from build123d import *

# Parameters (mm, degrees)
BOSS_EXTRU_1_DEPTH                  = 60
CHANFREIN2_SIZE                     = 10
CHANFREIN2_SIZE2                    = 20
CHANFREIN3_SIZE                     = 20
CHANFREIN3_SIZE2                    = 10
CONG_3_R                            = 2
ENL_V_MAT_EXTRU_4_DEPTH             = 2
ENL_V_MAT_EXTRU_4_DEPTH_BACK        = 66.720872054
ENL_V_MAT_EXTRU_4_START             = -4
ESQUISSE5_R                         = 16.05
ESQUISSE2_R                         = 1.7
ESQUISSE2_R_2                       = 10.1
ENL_V_MAT_EXTRU_1_DEPTH             = 70.720872183
ESQUISSE3_R                         = 1.6
ENL_V_MAT_EXTRU_2_DEPTH             = 78.097341186
ENL_V_MAT_EXTRU_5_REACH             = 71.721
ESQUISSE6_R                         = 3.25
ENL_V_MAT_EXTRU_5_DIRECTION_2_REACH = 71.721
CHANFREIN1_SIZE                     = 10
BOSS_EXTRU_3_REACH                  = 79.097
ESQUISSE8_W                         = 1.2
ESQUISSE8_H                         = 30
CONG_2_R                            = 2


with BuildPart() as part:
    # Esquisse1 → Boss.-Extru.1 (new body)
    with BuildSketch(Plane(origin=(0, 0, 0), x_dir=(0, 0, -1), z_dir=(1, 0, 0))):
        Polygon((0, -19), (0, 19), (30, 19), (30, 15), (4, 15), (4, -15), (30, -15), (30, -19), align=None)
    extrude(amount=BOSS_EXTRU_1_DEPTH)

    # Chanfrein2
    chanfrein2_edges = [part.edges().sort_by_distance(p)[0] for p in [
        (30, 15, -4),
    ]]
    chanfrein2_side = [part.faces().sort_by_distance(p)[0] for p in [
        (30, 0, -4),
    ]]
    chamfer(chanfrein2_edges, length=CHANFREIN2_SIZE, length2=CHANFREIN2_SIZE2, reference=chanfrein2_side[0])

    # Chanfrein3
    chanfrein3_edges = [part.edges().sort_by_distance(p)[0] for p in [
        (30, -15, -4),
    ]]
    chanfrein3_side = [part.faces().sort_by_distance(p)[0] for p in [
        (30, -15, -17),
    ]]
    chamfer(chanfrein3_edges, length=CHANFREIN3_SIZE, length2=CHANFREIN3_SIZE2, reference=chanfrein3_side[0])

    # Congé3
    cong_3_edges = [part.edges().sort_by_distance(p)[0] for p in [
        (30, 5, -4),
        (30, -5, -4),
    ]]
    fillet(cong_3_edges, radius=CONG_3_R)

    # Esquisse5 → Enlèv. mat.-Extru.4 (cut, two sides: drawn at the far end of the back side and taken through both)
    with BuildSketch(Plane.XY.offset(ENL_V_MAT_EXTRU_4_START - ENL_V_MAT_EXTRU_4_DEPTH_BACK)):
        with Locations(Location((30, 0, 0), (0, 0, 193.562911562))):
            Circle(ESQUISSE5_R)
    extrude(amount=ENL_V_MAT_EXTRU_4_DEPTH + ENL_V_MAT_EXTRU_4_DEPTH_BACK, mode=Mode.SUBTRACT)

    # Esquisse2 → Enlèv. mat.-Extru.1 (cut, through all)
    with BuildSketch(Plane.XY):
        with Locations((30, 13)):
            Circle(ESQUISSE2_R)
        with Locations((43, 0)):
            Circle(ESQUISSE2_R)
        with Locations((30, -13)):
            Circle(ESQUISSE2_R)
        with Locations((17, 0)):
            Circle(ESQUISSE2_R)
        with Locations((30, 0)):
            Circle(ESQUISSE2_R_2)
    extrude(amount=-ENL_V_MAT_EXTRU_1_DEPTH, mode=Mode.SUBTRACT)

    # Esquisse3 → Enlèv. mat.-Extru.2 (cut, through all)
    with BuildSketch(Plane.XZ.offset(19)):
        with Locations(Location((10, -15, 0), (0, 0, 270))):
            Circle(ESQUISSE3_R)
        with Locations(Location((50, -15, 0), (0, 0, 270))):
            Circle(ESQUISSE3_R)
    extrude(amount=-ENL_V_MAT_EXTRU_2_DEPTH, mode=Mode.SUBTRACT)

    # Enlèv. mat.-Extru.5: up to this face of the body (flat: up to its plane)
    enl_v_mat_extru_5_end = Plane(part.part.faces().sort_by_distance((30, -19, -15))[0])
    # Esquisse6 → Enlèv. mat.-Extru.5 (cut, up to the picked face)
    with BuildSketch(Plane(origin=(0, 0, 0), x_dir=(1, 0, 0), z_dir=(0, 1, 0)), mode=Mode.PRIVATE) as enl_v_mat_extru_5_sk1:
        with Locations(Location((10, 15, 0), (0, 0, 90))):
            Circle(ESQUISSE6_R)
    enl_v_mat_extru_5_tool1 = split(extrude(enl_v_mat_extru_5_sk1.sketch, amount=-ENL_V_MAT_EXTRU_5_REACH, mode=Mode.PRIVATE), bisect_by=enl_v_mat_extru_5_end, keep=Keep.BOTH, mode=Mode.PRIVATE)
    # Esquisse6 → Enlèv. mat.-Extru.5 (cut, up to the picked face)
    with BuildSketch(Plane(origin=(0, 0, 0), x_dir=(1, 0, 0), z_dir=(0, 1, 0)), mode=Mode.PRIVATE) as enl_v_mat_extru_5_sk2:
        with Locations(Location((50, 15, 0), (0, 0, 270))):
            Circle(ESQUISSE6_R)
    enl_v_mat_extru_5_tool2 = split(extrude(enl_v_mat_extru_5_sk2.sketch, amount=-ENL_V_MAT_EXTRU_5_REACH, mode=Mode.PRIVATE), bisect_by=enl_v_mat_extru_5_end, keep=Keep.BOTH, mode=Mode.PRIVATE)
    add(enl_v_mat_extru_5_tool1.solids().sort_by(Axis((10, 0, -15), (0, -1, 0)))[0], mode=Mode.SUBTRACT)
    add(enl_v_mat_extru_5_tool2.solids().sort_by(Axis((50, 0, -15), (0, -1, 0)))[0], mode=Mode.SUBTRACT)

    # Enlèv. mat.-Extru.5 direction 2: up to this face of the body (flat: up to its plane)
    enl_v_mat_extru_5_direction_2_end = Plane(part.part.faces().sort_by_distance((30, 19, -15))[0])
    # Esquisse6 → Enlèv. mat.-Extru.5 direction 2 (cut, up to the picked face)
    with BuildSketch(Plane(origin=(0, 0, 0), x_dir=(1, 0, 0), z_dir=(0, 1, 0)), mode=Mode.PRIVATE) as enl_v_mat_extru_5_direction_2_sk1:
        with Locations(Location((10, 15, 0), (0, 0, 90))):
            Circle(ESQUISSE6_R)
    enl_v_mat_extru_5_direction_2_tool1 = split(extrude(enl_v_mat_extru_5_direction_2_sk1.sketch, amount=ENL_V_MAT_EXTRU_5_DIRECTION_2_REACH, mode=Mode.PRIVATE), bisect_by=enl_v_mat_extru_5_direction_2_end, keep=Keep.BOTH, mode=Mode.PRIVATE)
    # Esquisse6 → Enlèv. mat.-Extru.5 direction 2 (cut, up to the picked face)
    with BuildSketch(Plane(origin=(0, 0, 0), x_dir=(1, 0, 0), z_dir=(0, 1, 0)), mode=Mode.PRIVATE) as enl_v_mat_extru_5_direction_2_sk2:
        with Locations(Location((50, 15, 0), (0, 0, 270))):
            Circle(ESQUISSE6_R)
    enl_v_mat_extru_5_direction_2_tool2 = split(extrude(enl_v_mat_extru_5_direction_2_sk2.sketch, amount=ENL_V_MAT_EXTRU_5_DIRECTION_2_REACH, mode=Mode.PRIVATE), bisect_by=enl_v_mat_extru_5_direction_2_end, keep=Keep.BOTH, mode=Mode.PRIVATE)
    add(enl_v_mat_extru_5_direction_2_tool1.solids().sort_by(Axis((10, 0, -15), (0, 1, 0)))[0], mode=Mode.SUBTRACT)
    add(enl_v_mat_extru_5_direction_2_tool2.solids().sort_by(Axis((50, 0, -15), (0, 1, 0)))[0], mode=Mode.SUBTRACT)

    # Chanfrein1
    # the kernel refuses this chamfer: 10 mm, written as the material it takes off along each edge
    with BuildSketch(Plane(origin=(0, -44.71682988, 0), x_dir=(-0.027495876610586372, 0, -0.9996219169112968), z_dir=(0, 1, 0))) as chanfrein1_piece_1:
        Polygon((CHANFREIN1_SIZE * 0.999621916911, -CHANFREIN1_SIZE * 0.0274958766106), (-CHANFREIN1_SIZE * 0.0274958766106, -CHANFREIN1_SIZE * 0.999621916911), (0, 0), align=None)
    extrude(amount=89.433659759, mode=Mode.SUBTRACT)

    # Boss.-Extru.3: up to this face of the body (flat: up to its plane)
    boss_extru_3_end = Plane(part.part.faces().sort_by_distance((30.791937825, -19, -15.346472798))[0])
    # Esquisse8 → Boss.-Extru.3 (add, up to the picked face)
    with BuildSketch(Plane(origin=(0, 19, 0), x_dir=(1, 0, 0), z_dir=(0, 1, 0)), mode=Mode.PRIVATE) as boss_extru_3_sk1:
        with Locations((59.4, 15)):
            Rectangle(ESQUISSE8_W, ESQUISSE8_H)
    boss_extru_3_tool1 = split(extrude(boss_extru_3_sk1.sketch, amount=-BOSS_EXTRU_3_REACH, mode=Mode.PRIVATE), bisect_by=boss_extru_3_end, keep=Keep.BOTH, mode=Mode.PRIVATE)
    # Esquisse8 → Boss.-Extru.3 (add, up to the picked face)
    with BuildSketch(Plane(origin=(0, 19, 0), x_dir=(1, 0, 0), z_dir=(0, 1, 0)), mode=Mode.PRIVATE) as boss_extru_3_sk2:
        Polygon((1.2, 30), (1.2, 10.497056275), (10.848528137, 0.848528137), (10, 0), (0, 10), (0, 30), align=None)
    boss_extru_3_tool2 = split(extrude(boss_extru_3_sk2.sketch, amount=-BOSS_EXTRU_3_REACH, mode=Mode.PRIVATE), bisect_by=boss_extru_3_end, keep=Keep.BOTH, mode=Mode.PRIVATE)
    add(boss_extru_3_tool1.solids().sort_by(Axis((59.4, 19, -15), (0, -1, 0)))[0])
    add(boss_extru_3_tool2.solids().sort_by(Axis((0.880987, 19, -20.248528), (0, -1, 0)))[0])

    # Congé2
    cong_2_edges = [part.edges().sort_by_distance(p)[0] for p in [
        (10, 0, 0),
        (0, 0, -10),
    ]]
    fillet(cong_2_edges, radius=CONG_2_R)


solid = part.part
Could you check a few things on this model? Use its own coordinates, in mm. A direction names the side the tool comes from. Give positions to 0.01 mm unless a question says otherwise; leave off trailing zeros. Order: outer loops, then holes, each group sorted by start corner. A loop starts at its lowest first (then second) coordinate and runs counter-clockwise, first axis right, second up. Notation, with made-up numbers: M -6,49.25 L 48,49.25 A16 ccw 48,57.25 Z; hole C -20.5,16.5 d2. An arc over 180 degrees is marked long. One line per question, with ' | ' between items.
1. I'm going to push flat-ended pins straight in: pin 1 (2 mm diameter, centred on x = 40.5, y = -5, fed in from -Z); pin 2 (1.5 mm diameter, centred on y = 11.5, z = -8, fed in from -X); pin 3 (6 mm diameter, centred on x = 50, z = -15, fed in from -Y); pin 4 (5.5 mm diameter, centred on x = 11, y = -1.5, fed in from -Z). Where does each tip first touch, or does it pass through?
Results:
pin 1: z = -2 | pin 2: x = 1.25 | pin 3: through | pin 4: z = -4.06
2. If I drill on line 1 (X direction, y = -16.5, z = -15); line 2 (Y direction, x = 17, z = -1); line 3 (Y direction, x = 38, z = -24), over which ranges is the centre line in solid material (lowest first)?
Results:
line 1: 0 to 6.75, 13.25 to 46.75, 53.25 to 60 | line 2: -19 to -1.7, 1.7 to 19 | line 3: -19 to -15, 15 to 19
3. We'd pull the mould along Z, two halves only. Please class faces 3 (the face through (58.8, 0, -20)), 4 (the face through (48.755, -14.992, -11.998)), 5 (the face through (10.07, 0.27, -0.15)): +Z half, -Z half, draft (parallel to the pull), parting line (faces both ways), or undercut.
Results:
face 3: draft | face 4: undercut | face 5: +Z half
4. I want a section at D-D (z = -3). List the corners of the cut face in (x, y) for me.
Results:
outline: M 7,-19 L 60,-19 L 60,19 L 7,19 Z; hole C 30,0 d32.1
5. I want a section at C-C (y = 13). List the corners of the cut face in (x, z) for me, and give its area (3 significant figures).
Results:
outline: M 0,-30 L 1.2,-30 L 1.2,-20 L 20.59,-20 L 20.59,-2 L 28.3,-2 L 28.3,0 L 10.83,0 A2 ccw 9.41,-0.59 L 0.59,-9.41 A2 ccw 0,-10.83 Z; M 31.7,-2 L 39.41,-2 L 39.41,-20 L 58.8,-20 L 58.8,-30 L 60,-30 L 60,0 L 31.7,0 Z; hole C 10,-15 d6.5; hole C 50,-15 d6.5 | area: 762 mm²
6. For faces 1 (the face through (41.65, -1.03, -0.99)), 2 (the face through (52.03, -4.8, -4.29)), which set-ups out of +Z, -Z, +X, -X, +Y, -Y let a thin tool reach every point of the face, with its end or its side?
Results:
face 1: +Z, -Z | face 2: -Z
7. I want a section at B-B (y = 0). List the corners of the cut face in (x, z) for me, and give its area (3 significant figures).
Results:
outline: M 0,-30 L 1.2,-30 L 1.2,-10.5 L 7.7,-4 L 13.95,-4 L 13.95,-2 L 15.3,-2 L 15.3,0 L 10.83,0 A2 ccw 9.41,-0.59 L 0.59,-9.41 A2 ccw 0,-10.83 Z; M 18.7,-2 L 19.9,-2 L 19.9,0 L 18.7,0 Z; M 40.1,-2 L 41.3,-2 L 41.3,0 L 40.1,0 Z; M 44.7,-2 L 46.05,-2 L 46.05,-4 L 58.8,-4 L 58.8,-30 L 60,-30 L 60,0 L 44.7,0 Z | area: 155 mm²
8. I want a section at A-A (x = 30). List the corners of the cut face in (y, z) for me, and give its area (3 significant figures).
Results:
outline: M -19,-30 L -16.05,-30 L -16.05,-2 L -14.7,-2 L -14.7,0 L -19,0 Z; M -11.3,-2 L -10.1,-2 L -10.1,0 L -11.3,0 Z; M 10.1,-2 L 11.3,-2 L 11.3,0 L 10.1,0 Z; M 14.7,-2 L 16.05,-2 L 16.05,-30 L 19,-30 L 19,0 L 14.7,0 Z | area: 187 mm²
